The drawing under review shows one solid part. Ordinate dimensions are in mm from its lowest x, y, z. A direction names the side the tool comes from. Coordinates: 2 decimals unless noted, no trailing zeros. Write each loop counter-clockwise with the first axis right and the second up, starting at its lowest first coordinate (ties: lowest second). Pieces come first, ordered by that corner, then holes.
Q1. Add section D-D, the plane x = 1. Give the boundary of the cut face in (y, z).
Q2. Add section C-C, the plane z = 1.85. Give the boundary of the cut face in (x, y) (3 decimals).
Q3. The part is to be moulded in two halves that separate along Y. For the marked faces 1, 2, 3 and 4, say which applies: +Y half, -Y half, draft (parallel to the pull), parting line (faces both ways), or undercut.
Q4. Clearance check with a flat-ended pin moving along its axis: pin 1 Ø1.8 at (x, y) = (4.5, 4.5) entering from -Z. State where the tip first meets the part, or that it passes through.
Q5. Machinability: for the marked faces 5 and 6, which of the approach directions +Z, -Z, +X, -X, +Y, -Y give a long, thin tool a straight path to every point of the face, cutting with its end or side? Answer none if there is none.
Q6. Add section A-A, the plane y = 14. Give the boundary of the cut face in (x, z) (3 decimals), plus the area to 4 significant figures.
Q7. To check wall thickness, follow probe 1 along Y at (x, z) = (4.5, 0.6); probe 2 along Y at (x, z) = (3.5, 2.55); probe 3 along X at (y, z) = (22.5, 1.95). State the ranges of each line that lie inside material, in increasing order.
Q8. Add section B-B, the plane x = 4.5. Give the boundary of the cut face in (y, z), plus the area to 3 significant figures.
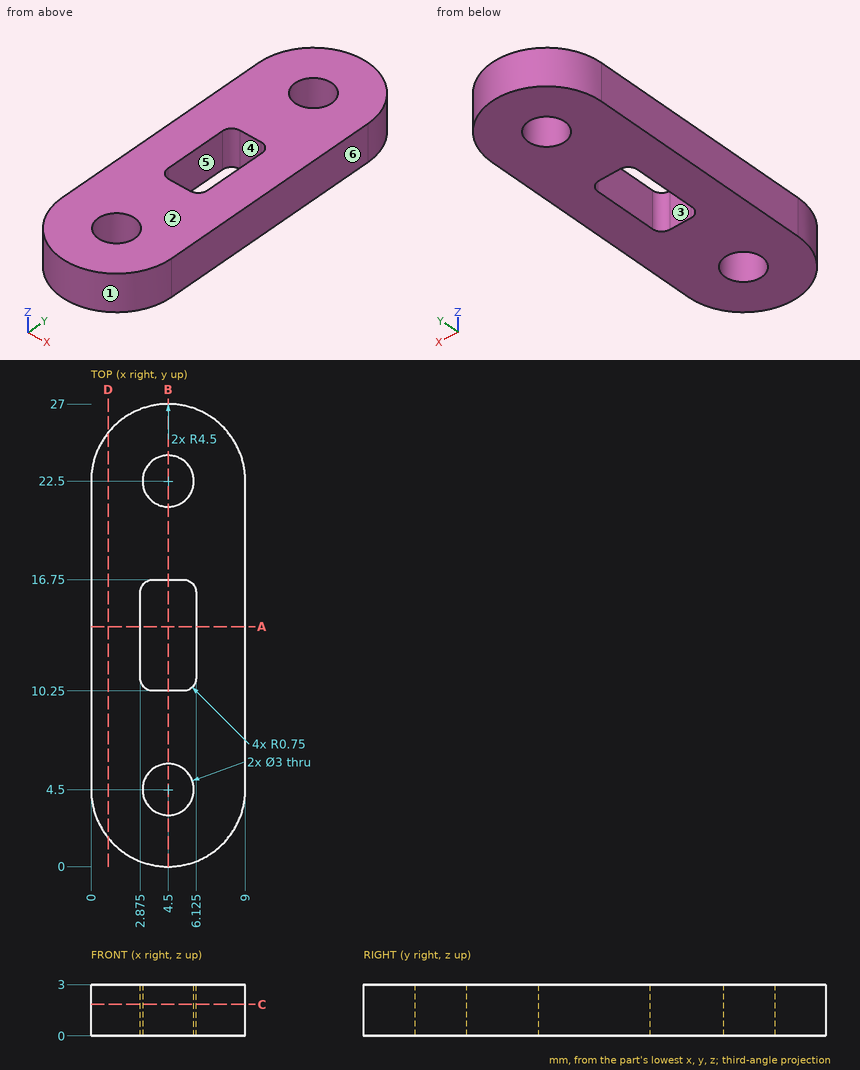
Here are the results:
1. outline: (1.67, 0) - (25.33, 0) - (25.33, 3) - (1.67, 3) - close
2. outline: (0, 4.5) arc R4.5 ccw to (9, 4.5) - (9, 22.5) arc R4.5 ccw to (0, 22.5) - close; hole (2.875, 11) arc R0.75 ccw to (3.625, 10.25) - (5.375, 10.25) arc R0.75 ccw to (6.125, 11) - (6.125, 16) arc R0.75 ccw to (5.375, 16.75) - (3.625, 16.75) arc R0.75 ccw to (2.875, 16) - close; hole circle Ø3 at (4.5, 4.5); hole circle Ø3 at (4.5, 22.5)
3. face 1: -Y half
3. face 2: draft
3. face 3: undercut
3. face 4: undercut
4. pin 1: passes through
5. face 5: +Z, -Z
5. face 6: +Z, -Z, +X, +Y, -Y
6. outline: (0, 0) - (2.875, 0) - (2.875, 3) - (0, 3) - close; (6.125, 0) - (9, 0) - (9, 3) - (6.125, 3) - close
6. area: 17.25 mm2
7. probe 1: y = 0 to 3, 6 to 10.25, 16.75 to 21, 24 to 27
7. probe 2: y = 0.11 to 3.38, 5.62 to 10.26, 16.74 to 21.38, 23.62 to 26.89
7. probe 3: x = 0 to 3, 6 to 9
8. outline: (0, 0) - (3, 0) - (3, 3) - (0, 3) - close; (6, 0) - (10.25, 0) - (10.25, 3) - (6, 3) - close; (16.75, 0) - (21, 0) - (21, 3) - (16.75, 3) - close; (24, 0) - (27, 0) - (27, 3) - (24, 3) - close
8. area: 43.5 mm2
